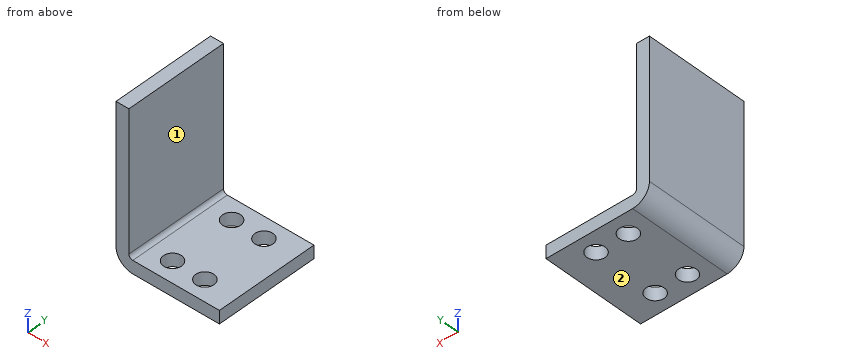
from build123d import *

# Parameters (mm, degrees)
F1_DEPTH = 40
F2_R     = 3
F3_R     = 13
F5_D     = 14


with BuildPart() as f1:
    # F0 (on Front) → F1 (new body, symmetric)
    with BuildSketch(Plane.XZ):
        Polygon((10, 120), (0, 120), (0, 0), (80, 0), (80, 10), (10, 10), align=None)
    extrude(amount=F1_DEPTH, both=True)

    # F2
    f2_edges = [f1.edges().sort_by_distance(p)[0] for p in [
        (10, 0, 10),
    ]]
    fillet(f2_edges, radius=F2_R)

    # F3
    f3_edges = [f1.edges().sort_by_distance(p)[0] for p in [
        (0, 0, 0),
    ]]
    fillet(f3_edges, radius=F3_R)

    # F5 (through all)
    with Locations(Plane.XY.offset(10)):
        with Locations((55, 25), (55, -25), (30, -25), (30, 25)):
            Hole(F5_D / 2)


solid = f1.part
Input: part model. Units: mm. Frame: model coordinates. Face numbers are marked on the shaded views. A direction names the side the tool comes from. Give positions to 0.01 mm unless a question says otherwise; leave off trailing zeros. Order: outer loops, then holes, each group sorted by start corner. A loop starts at its lowest first (then second) coordinate and runs counter-clockwise, first axis right, second up. Notation, with made-up numbers: M 65,75.25 L 70,75.25 A13 ccw 70,92.25 Z; hole C 22,-12.5 d11. An arc over 180 degrees is marked long. Answer as a JSON object with one key per item and string values.
1. Cut plane A-A, the plane y = 25. Output: boundary loops of the cut face in (x, z).
Result sheet:
{"outline": "M 0,13 A13 ccw 13,0 L 23,0 L 23,10 L 13,10 A3 cw 10,13 L 10,120 L 0,120 Z; M 37,0 L 48,0 L 48,10 L 37,10 Z; M 62,0 L 80,0 L 80,10 L 62,10 Z"}
2. First-contact query: P1, Ø16, axis at x = 30, y = -25, coming from the +Z side; P2, Ø24, axis at y = 12.5, z = 57, coming from the +X side; P3, Ø2, axis at x = 10.5, y = 2, coming from the -Z side. Flat tips, straight axial feed; report the tip coordinate or a pass-through.
Result sheet:
{"P1": "z = 10", "P2": "x = 10", "P3": "z = 0.09"}
3. Ray query, line 1 (Y direction, x = 55, z = 7); line 2 (Z direction, x = 29, y = -16). Return the intervals inside material, ascending. Write a range as [from, to].
Result sheet:
{"line 1": "[-40, -32], [-18, 18], [32, 40]", "line 2": "[0, 10]"}
4. Reachability of the marked faces 1 and 2 from +Z, -Z, +X, -X, +Y, -Y: full face, straight path, thin tool, end or side. Return the list, or none.
Result sheet:
{"face 1": "+Z, +X, +Y, -Y", "face 2": "-Z, +X, -X, +Y, -Y"}
5. Cut plane C-C, the plane y = 8. Output: boundary loops of the cut face in (x, z).
Result sheet:
{"outline": "M 0,13 A13 ccw 13,0 L 80,0 L 80,10 L 13,10 A3 cw 10,13 L 10,120 L 0,120 Z"}
6. Cut plane D-D, the plane z = 81. Output: boundary loops of the cut face in (x, y), and give its area (3 significant figures).
Result sheet:
{"outline": "M 0,-40 L 10,-40 L 10,40 L 0,40 Z", "area": "800 mm²"}
7. Cut plane B-B, the plane x = 55. Output: boundary loops of the cut face in (y, z).
Result sheet:
{"outline": "M -40,0 L -32,0 L -32,10 L -40,10 Z; M -18,0 L 18,0 L 18,10 L -18,10 Z; M 32,0 L 40,0 L 40,10 L 32,10 Z"}
